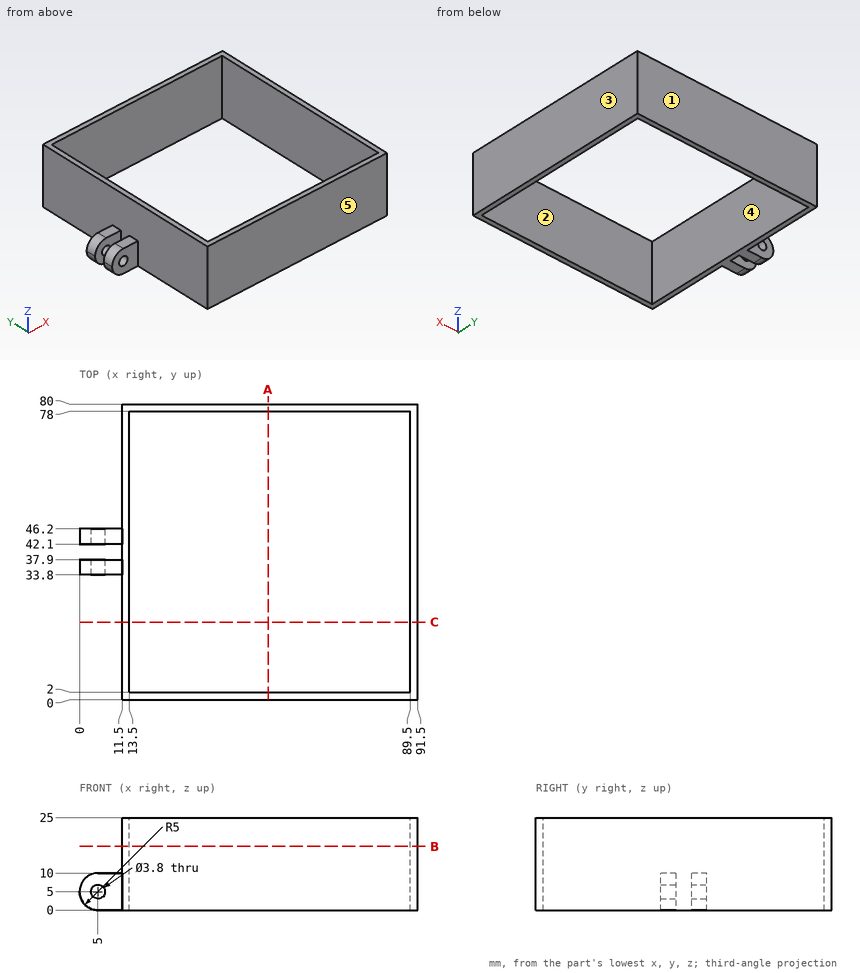
For this review, use the dimensioned drawing (mm, ordinates from the lowest corner) and the shaded views. A direction names the side the tool comes from. Coordinates: 2 decimals unless noted, no trailing zeros. Order: outer loops, then holes, each group sorted by start corner. A loop starts at its lowest first (then second) coordinate and runs counter-clockwise, first axis right, second up. Notation, with made-up numbers: (87, 54.5) - (91, 54.5) arc R22 ccw to (91, 87.5) - close; hole circle Ø1 at (68.5, 86.25). An arc over 180 degrees is marked (long way). Answer in a Markdown table with one row per item.
(1) Consider section B-B on z = 17.25. State the section outline as (x, y) points, plus the area to 3 significant figures.
Checked values:
| item | result |
|---|---|
| outline | (11.5, 0) - (91.5, 0) - (91.5, 80) - (11.5, 80) - close; hole (13.5, 2) - (89.5, 2) - (89.5, 78) - (13.5, 78) - close |
| area | 624 mm^2 |
(2) Clearance check with flat-ended pins moving along their axes: pin 1 (4.5 mm diameter, centred on x = 7, y = 43.5, fed in from +Z); pin 2 (8 mm diameter, centred on y = 52, z = 21, fed in from -X); pin 3 (11 mm diameter, centred on x = 3, z = 7.5, fed in from -Y). State where each tip first meets the part, or that it passes through.
Checked values:
| item | result |
|---|---|
| pin 1 | z = 10 |
| pin 2 | x = 11.5 |
| pin 3 | y = 33.8 |
(3) The part is to be moulded in two halves that separate along X. For the marked faces 1, 2 and 3, say which applies: released by +X, released by -X, zero draft, split by the parting line, or undercut.
Checked values:
| item | result |
|---|---|
| face 1 | zero draft |
| face 2 | undercut |
| face 3 | released by +X |
(4) Wall thickness on line 1 along Y through (x, z) = (25, 1.5); line 2 along X through (y, z) = (36.5, 11.25); line 3 along Z through (x, y) = (5, 44): over which ranges is each line inside the solid? List them lowest first. Write a range as from..to.
Checked values:
| item | result |
|---|---|
| line 1 | 0..2, 78..80 |
| line 2 | 11.5..13.5, 89.5..91.5 |
| line 3 | 0..3.1, 6.9..10 |
(5) Consider section A-A on x = 51. State the section outline as (y, z) points.
Checked values:
| item | result |
|---|---|
| outline | (0, 0) - (2, 0) - (2, 25) - (0, 25) - close; (78, 0) - (80, 0) - (80, 25) - (78, 25) - close |
(6) Consider section C-C on y = 21. State the section outline as (x, z) points.
Checked values:
| item | result |
|---|---|
| outline | (11.5, 0) - (13.5, 0) - (13.5, 25) - (11.5, 25) - close; (89.5, 0) - (91.5, 0) - (91.5, 25) - (89.5, 25) - close |
(7) For the marked faces 4 and 5, list the 3-axis set-ups (+Z, -Z, +X, -X, +Y, -Y) from which the entire face can be reached by the end or side of a thin tool; tool diameter is ignored.
Checked values:
| item | result |
|---|---|
| face 4 | +Z, -Z |
| face 5 | +Z, -Z, +X, -X, -Y |
